Can you work these out from the model? Positions are in its coordinate system, mm. A direction names the side the tool comes from. Give positions to 0.01 mm unless a question says otherwise; leave off trailing zeros. Order: outer loops, then holes, each group sorted by start corner. A loop starts at its lowest first (then second) coordinate and runs counter-clockwise, first axis right, second up. Notation, with made-up numbers: (-16.5, 75) - (38.5, 75) arc R20 ccw to (38.5, 96) - close; hole circle Ø2 at (66, -17.5). An arc over 180 degrees is marked (long way). Answer as a JSON object with one key per item and string values.
```python
from build123d import *

# Parameters (mm, degrees)
SKETCH2_R           = 50
SKETCH2_R_2         = 15
BOSS_EXTRUDE1_DEPTH = 25
BOSS_EXTRUDE2_START = -75
BOSS_EXTRUDE2_DEPTH = 75
SKETCH4_R           = 5
BOSS_EXTRUDE3_DEPTH = 60


with BuildPart() as part:
    # Sketch2 → Boss-Extrude1 (new body)
    with BuildSketch(Plane(origin=(0, 0, 0), x_dir=(1, 0, 0), z_dir=(0, 1, 0))):
        with Locations(Location((0, 0, 0), (0, 0, 270))):
            Circle(SKETCH2_R)
        with Locations(Location((0, 0, 0), (0, 0, 270))):
            Circle(SKETCH2_R_2, mode=Mode.SUBTRACT)
    extrude(amount=BOSS_EXTRUDE1_DEPTH)

    # Sketch3 → Boss-Extrude2 (add)
    with BuildSketch(Plane(origin=(0, 25, 0), x_dir=(1, 0, 0), z_dir=(0, 1, 0)).offset(BOSS_EXTRUDE2_START)):
        with BuildLine():
            Line((47.696960071, 15), (60, 15))
            Line((60, 15), (60, -15))
            Line((60, -15), (47.696960071, -15))
            ThreePointArc((47.696960071, -15), (50, 0), (47.696960071, 15))
        make_face()
    extrude(amount=BOSS_EXTRUDE2_DEPTH)

    # Sketch4 → Boss-Extrude3 (add)
    with BuildSketch(Plane(origin=(60, 0, 0), x_dir=(0, 0, -1), z_dir=(1, 0, 0))):
        with Locations((0, -50)):
            Circle(SKETCH4_R)
    extrude(amount=-BOSS_EXTRUDE3_DEPTH)


solid = part.part
```
Q1. If we section it at B-B, the plane x = 10: Please give me the cut outline in (y, z).
Recorded:
{"outline": "circle Ø10 at (-50, 0); (0, -48.99) - (25, -48.99) - (25, -11.18) - (0, -11.18) - close; (0, 11.18) - (25, 11.18) - (25, 48.99) - (0, 48.99) - close"}
Q2. If we section it at C-C, the plane y = 6.5: Please give me the cut outline in (x, z).
Recorded:
{"outline": "(47.7, -15) - (60, -15) - (60, 15) - (47.7, 15) arc R50 ccw (long way) to start; hole circle Ø30 at (0, 0)"}
Q3. I'm going to push flat-ended pins straight in: pin 1 Ø5 at (x, z) = (-0.5, 18) entering from -Y; pin 2 Ø3.5 at (x, y) = (56, -30) entering from -Z; pin 3 Ø8 at (y, z) = (-52.5, -0.5) entering from -X. Where does each tip first touch, or does it pass through?
Recorded:
{"pin 1": "stops at y = 0", "pin 2": "stops at z = -15", "pin 3": "stops at x = 0"}
Q4. If we section it at D-D, the plane x = 24.5: Please give me the cut outline in (y, z).
Recorded:
{"outline": "circle Ø10 at (-50, 0); (0, -43.59) - (25, -43.59) - (25, 43.59) - (0, 43.59) - close"}
Q5. I need wall thicknesses on L1, parallel to X at y = 15, z = 0; L2, parallel to X at y = -16, z = 0.5; L3, parallel to Y at x = -19, z = 1.5. Which ranges of each line are inside material? Lowest first, please.
Recorded:
{"L1": "x = -50 to -15, 15 to 60", "L2": "x = 50 to 60", "L3": "y = 0 to 25"}
Q6. Which directions (+Z, -Z, +X, -X, +Y, -Y) give clear straight access to the entire face, cutting with the end or side of a thin tool? Please do faces 5 (the face through (30.42, -54.88, 1.08)), 6 (the face through (-49.96, 12.32, -1.99)), 7 (the face through (54, -50, -10)), 8 (the face through (54, -13, 15)).
Recorded:
{"face 5": "-X", "face 6": "+Y, -Y", "face 7": "-Z, +X, -X, -Y", "face 8": "+Z, +X, +Y, -Y"}
Q7. If we section it at A-A, the plane z = 0: Please give me the cut outline in (x, y), then the cut area to 3 significant figures.
Recorded:
{"outline": "(-50, 0) - (-15, 0) - (-15, 25) - (-50, 25) - close; (0, -55) - (60, -55) - (60, 25) - (15, 25) - (15, 0) - (50, 0) - (50, -45) - (0, -45) - close", "area": "3,050 mm^2"}
Q8. We'd pull the mould along Z, two halves only. Please class faces 1 (the face through (54, -50, 10)), 2 (the face through (54, -13, -15)), 3 (the face through (50, -25, 0)), 4 (the face through (0.66, 12.325, -14.985)): released by +Z, released by -Z, zero draft, split by the parting line, or undercut.
Recorded:
{"face 1": "zero draft", "face 2": "released by -Z", "face 3": "undercut", "face 4": "undercut"}
